The listing builds one solid part. Answer for the finished solid, in the listing's coordinates (mm). Round coordinates to 2 decimals unless told otherwise and drop trailing zeros. Order: outer loops, then holes, each group sorted by start corner. A loop starts at its lowest first (then second) coordinate and runs counter-clockwise, first axis right, second up. Notation, with made-up numbers: (29, 68.25) -> (52, 68.25) arc R29 cw to (52, 101.25) -> close; hole circle Ø8 at (6.25, 62). An arc over 180 degrees is marked (long way). Return JSON: item names as keys, results as strings. Group by question number.
(1) The part is cut by section A-A (z = 0). Determine the outline of the cut face in (x, y), plus the area to 3 significant figures.
(2) The part is cut by section B-B (z = 23). Determine the outline of the cut face in (x, y).
(3) Determine the mould class of faces 1 (the face through (20, -25.4, 1)), 2 (the face through (31.63, -12.88, 36.76)), 3 (the face through (22.52, -12.88, -27.93)) for opening direction X: +X half, -X half, draft (parallel to the pull), parting line (faces both ways), or undercut.
(4) The part is cut by section C-C (y = -11.75). Count the separate pieces of the cut face and the enclosed holes in it, plus the area to 3 significant figures.
(5) Consider line 1 (X direction, y = -19.5, z = 31); line 2 (Z direction, x = 3, y = -13.75); line 3 (X direction, y = -18.5, z = -1.5). Determine where each line is inside the solid, lowest interval first. Write a range as [from, to].
(6) Each of these flat-tipped pins is pushed along its axis until it touches: pin 1 (10.5 mm diameter, centred on x = 38, y = -10.5, fed in from +Z); pin 2 (12 mm diameter, centred on x = -45.5, y = -4, fed in from +Z); pin 3 (5 mm diameter, centred on x = 21, y = -10, fed in from -Z). Where does it stop, or does it pass through?
(7) The part is cut by section D-D (z = -74). Determine the outline of the cut face in (x, y).
from build123d import *

# Parameters (mm, degrees)
F0_R     = 93.98
F1_DEPTH = 25.4
F2_W     = 9.525
F2_H     = 25.4
F2_R     = 1.905
F3_DEPTH = 25.401
F5_DEPTH = 25.401
F7_DEPTH = 25.401


with BuildPart() as f1:
    # F0 (on Front) → F1 (new body)
    with BuildSketch(Plane.XZ):
        Circle(F0_R)
    extrude(amount=F1_DEPTH)

    # F2 (on Front) → F3 (cut, through all)
    with BuildSketch(Plane.XZ):
        Rectangle(F2_W, F2_H)
        with Locations((0, 30.1752)):
            Circle(F2_R)
        with Locations((0, -30.1752)):
            Circle(F2_R)
    extrude(amount=F3_DEPTH, mode=Mode.SUBTRACT)

    # F4 (on face) → F5 (cut, through all)
    with BuildSketch(Plane.XZ.offset(25.4)):
        with BuildLine():
            ThreePointArc((-55.5625, 12.7), (0, 56.995451), (55.5625, 12.7))
            Line((55.5625, 12.7), (78.498342, 12.7))
            ThreePointArc((78.498342, 12.7), (0, 79.519053), (-78.498342, 12.7))
            Line((-78.498342, 12.7), (-55.5625, 12.7))
        make_face()
        with BuildLine():
            Line((78.498342, -12.7), (55.5625, -12.7))
            ThreePointArc((55.5625, -12.7), (0, -56.995451), (-55.5625, -12.7))
            Line((-55.5625, -12.7), (-78.498342, -12.7))
            ThreePointArc((-78.498342, -12.7), (0, -79.519053), (78.498342, -12.7))
        make_face()
    extrude(amount=-F5_DEPTH, mode=Mode.SUBTRACT)

    # F6 (on face) → F7 (cut, through all)
    with BuildSketch(Plane.XZ.offset(25.4)):
        with BuildLine():
            ThreePointArc((-33.554508, 12.7), (-22.309038, 28.098075), (-4.7625, 35.56))
            Line((-4.7625, 35.56), (-4.7625, 48.26))
            ThreePointArc((-4.7625, 48.26), (-31.318534, 37.025106), (-46.801912, 12.7))
            Line((-46.801912, 12.7), (-33.554508, 12.7))
        make_face()
        with BuildLine():
            Line((4.7625, 48.26), (4.7625, 35.56))
            ThreePointArc((4.7625, 35.56), (22.309038, 28.098075), (33.554508, 12.7))
            Line((33.554508, 12.7), (46.801912, 12.7))
            ThreePointArc((46.801912, 12.7), (31.318534, 37.025106), (4.7625, 48.26))
        make_face()
        with BuildLine():
            ThreePointArc((4.7625, -48.26), (31.318534, -37.025106), (46.801912, -12.7))
            Line((46.801912, -12.7), (33.554508, -12.7))
            ThreePointArc((33.554508, -12.7), (22.309038, -28.098075), (4.7625, -35.56))
            Line((4.7625, -35.56), (4.7625, -48.26))
        make_face()
        with BuildLine():
            Line((-4.7625, -48.26), (-4.7625, -35.56))
            ThreePointArc((-4.7625, -35.56), (-22.309038, -28.098075), (-33.554508, -12.7))
            Line((-33.554508, -12.7), (-46.801912, -12.7))
            ThreePointArc((-46.801912, -12.7), (-31.318534, -37.025106), (-4.7625, -48.26))
        make_face()
    extrude(amount=-F7_DEPTH, mode=Mode.SUBTRACT)


solid = f1.part
Answer below:
{
 "1": {"outline": "(-93.98, -25.4) -> (-4.76, -25.4) -> (-4.76, 0) -> (-93.98, 0) -> close; (4.76, -25.4) -> (93.98, -25.4) -> (93.98, 0) -> (4.76, 0) -> close", "area": "4,530 mm²"},
 "2": {"outline": "(-91.12, -25.4) -> (-76.12, -25.4) -> (-76.12, 0) -> (-91.12, 0) -> close; (-52.15, -25.4) -> (-42.69, -25.4) -> (-42.69, 0) -> (-52.15, 0) -> close; (-27.54, -25.4) -> (27.54, -25.4) -> (27.54, 0) -> (-27.54, 0) -> close; (42.69, -25.4) -> (52.15, -25.4) -> (52.15, 0) -> (42.69, 0) -> close; (76.12, -25.4) -> (91.12, -25.4) -> (91.12, 0) -> (76.12, 0) -> close"},
 "3": {"face 1": "draft", "face 2": "undercut", "face 3": "undercut"},
 "4": {"separate pieces": "1", "enclosed holes": "9", "area": "16,500 mm²"},
 "5": {"line 1": "x = [-88.72, -73.23], [-47.83, -37.29], [-18.06, -1.72], [1.72, 18.06], [37.29, 47.83], [73.23, 88.72]", "line 2": "z = [-93.93, -79.46], [-56.92, -12.7], [12.7, 56.92], [79.46, 93.93]", "line 3": "x = [-93.97, -4.76], [4.76, 93.97]"},
 "6": {"pin 1": "stops at z = 88.09", "pin 2": "stops at z = 85.28", "pin 3": "stops at z = -92.14"},
 "7": {"outline": "(-57.93, -25.4) -> (-29.11, -25.4) -> (-29.11, 0) -> (-57.93, 0) -> close; (29.11, -25.4) -> (57.93, -25.4) -> (57.93, 0) -> (29.11, 0) -> close"}
}
